Part model, mm, in its own coordinate system. A direction names the side the tool comes from. Round coordinates to 2 decimals unless told otherwise and drop trailing zeros. Order: outer loops, then holes, each group sorted by start corner. A loop starts at its lowest first (then second) coordinate and runs counter-clockwise, first axis right, second up. Notation, with made-up numbers: (51.5, -34) - (102.5, -34) arc R26 ccw to (102.5, -14) - close; hole circle Ø3 at (38.5, 38.5). An arc over 180 degrees is marked (long way). Answer as a JSON object with one key per item and string values.
```python
from build123d import *

# Parameters (mm, degrees)
F0_R      = 22.5
F1_DEPTH  = 143.8402
F2_R      = 13
F3_DEPTH  = 1.905
F4_R      = 6
F5_DEPTH  = 0.635
F6_R      = 5
F7_DEPTH  = 23.495
F10_DEPTH = 20.0499
F11_R     = 0.635
F12_DEPTH = 23.495
F13_R     = 1.5875
F14_DEPTH = 12.7
F15_SIZE  = 0.635


with BuildPart() as f1:
    # F0 (on Top) → F1 (new body)
    with BuildSketch(Plane.XY):
        Circle(F0_R)
    extrude(amount=-F1_DEPTH)

    # F2 (on face) → F3 (join)
    with BuildSketch(Plane(origin=(0, 0, -143.8402), x_dir=(1, 0, 0), z_dir=(0, 0, -1))):
        Circle(F2_R)
    extrude(amount=F3_DEPTH)

    # F4 (on face) → F5 (join)
    with BuildSketch(Plane(origin=(0, 0, -145.7452), x_dir=(1, 0, 0), z_dir=(0, 0, -1))):
        Circle(F4_R)
    extrude(amount=F5_DEPTH)

    # F6 (on face) → F7 (join)
    with BuildSketch(Plane(origin=(0, 0, -146.3802), x_dir=(1, 0, 0), z_dir=(0, 0, -1))):
        Circle(F6_R)
    extrude(amount=F7_DEPTH)

    # F9 (on offset) → F10 (cut, through all)
    with BuildSketch(Plane.XZ.offset(-2.4511)):
        with BuildLine():
            Line((-1.9812, -169.8752), (0, -169.8752))
            Line((0, -169.8752), (1.9812, -169.8752))
            Line((1.9812, -169.8752), (1.9812, -151.7396))
            ThreePointArc((1.9812, -151.7396), (0, -149.7584), (-1.9812, -151.7396))
            Line((-1.9812, -151.7396), (-1.9812, -169.8752))
        make_face()
    extrude(amount=-F10_DEPTH, mode=Mode.SUBTRACT)

    # F11 (on face) → F12 (cut)
    with BuildSketch(Plane(origin=(0, 0, -169.8752), x_dir=(1, 0, 0), z_dir=(0, 0, -1))):
        Circle(F11_R)
    extrude(amount=-F12_DEPTH, mode=Mode.SUBTRACT)

    # F13 (on face) → F14 (cut)
    with BuildSketch(Plane(origin=(0, 0, -143.8402), x_dir=(1, 0, 0), z_dir=(0, 0, -1))):
        with Locations((0, 17.375)):
            Circle(F13_R)
        with Locations((-17.375, 0)):
            Circle(F13_R)
        with Locations((0, -17.375)):
            Circle(F13_R)
        with Locations((17.375, 0)):
            Circle(F13_R)
    extrude(amount=-F14_DEPTH, mode=Mode.SUBTRACT)

    # F15
    f15_edges = [f1.edges().sort_by_distance(p)[0] for p in [
        (-0.635, 0, -169.8752),
        (-18.9625, 0, -143.8402),
        (-1.5875, 17.375, -143.8402),
        (15.7875, 0, -143.8402),
        (-1.5875, -17.375, -143.8402),
        (-2.74718, -4.177679, -169.8752),
        (-13, 0, -145.7452),
        (-22.5, 0, -143.8402),
    ]]
    chamfer(f15_edges, length=F15_SIZE)


solid = f1.part
```
Item 1: Probe L1, parallel to Y at x = 0, z = -134.5; L2, parallel to Y at x = 0, z = -161 (3 decimals); L3, parallel to Y at x = -11, z = -44. List the from-to ranges inside material, lowest first. Write a range as from..to.
Taken from the geometry:
{"L1": "-22.5..-18.96, -15.79..15.79, 18.96..22.5", "L2": "-5..-0.635, 0.635..2.451", "L3": "-19.63..19.63"}
Item 2: Tool access for faces 4 (the cylindrical face through (-10.316, 7.91, -144.466)), 5 (the flat face through (0, 2.451, -160)): list every direction of +Z, -Z, +X, -X, +Y, -Y with a clear straight run to the whole face (end or side of a thin tool).
Taken from the geometry:
{"face 4": "-Z", "face 5": "-Z, +Y"}
Item 3: Cut at A-A (z = -77). Write the cut outline in (x, y), plus the area to 3 significant figures.
Taken from the geometry:
{"outline": "circle Ø45 at (0, 0)", "area": "1,590 mm2"}
Item 4: Drop flat-ended pins along their axis: P1, Ø4, axis at x = -13.5, z = -17.5, coming from the +Y side; P2, Ø8, axis at y = -18, z = -59.5, coming from the +X side; P3, Ø2.5, axis at x = 18, y = -0.5, coming from the -Z side. Give the stop position or say it passes through.
Taken from the geometry:
{"P1": "y = 19.34", "P2": "x = 17.61", "P3": "z = -143.67"}
Item 5: Two-plate mould, pull along X, no slides. Class faces 1 (the cylindrical face through (10.382, -19.961, -70.6)), 2 (the flat face through (-17, 0, -131.14)), 3 (the flat face through (-1, -1.2, -169.875)): pulls with the +X half, pulls with the -X half, needs draft (parallel to the pull), parting line crosses it, or undercut.
Taken from the geometry:
{"face 1": "parting line crosses it", "face 2": "undercut", "face 3": "needs draft"}
